Read the model definition and answer for the solid it produces. Units are mm, in the model's axes. Coordinates: 2 decimals unless noted, no trailing zeros. Order: outer loops, then holes, each group sorted by start corner. A loop starts at its lowest first (then second) coordinate and runs counter-clockwise, first axis right, second up.
```python
from build123d import *

# Parameters (mm, degrees)
BOSS_EXTRUDE1_DEPTH             = 2.794
CUT_EXTRUDE1_DEPTH              = 89.482328967
CUT_EXTRUDE1_DEPTH_BACK         = 89.482328967
BOSS_EXTRUDE2_REACH             = 90.482
SKETCH3_W                       = 5.588
SKETCH3_H                       = 12.7
BOSS_EXTRUDE2_DIRECTION_2_REACH = 90.482
BOSS_EXTRUDE3_REACH             = 92.049
SKETCH4_R                       = 2.5273
BOSS_EXTRUDE3_DIRECTION_2_REACH = 92.049
SKETCH6_R                       = 1.2192
CUT_EXTRUDE8_DEPTH              = 91.178457469
CHAMFER1_SIZE                   = 3.175
CUT_EXTRUDE10_DEPTH             = 91.178457469


with BuildPart() as part:
    # Sketch1 → Boss-Extrude1 (new, symmetric)
    with BuildSketch(Plane.XY):
        Polygon((-6.06425, 85.600032), (22.225, 85.600032), (22.225, 0), (-22.225, 0), (-22.225, 85.600032), (-11.90625, 85.600032), (-11.90625, 53.850032), (-6.06425, 53.850032), align=None)
    extrude(amount=BOSS_EXTRUDE1_DEPTH, both=True)

    # Sketch2 → Cut-Extrude1 (cut, two sides: drawn at the far end of the back side and taken through both)
    with BuildSketch(Plane.XY.offset(-CUT_EXTRUDE1_DEPTH_BACK)):
        Polygon((-22.225, 27.78125), (-16.66875, 27.78125), (-16.66875, 30.1625), (-11.90625, 30.1625), (-11.90625, 27.78125), (-6.35, 27.78125), (-6.35, 23.01875), (-11.90625, 23.01875), (-11.90625, 20.6375), (-16.66875, 20.6375), (-16.66875, 23.01875), (-22.225, 23.01875), align=None)
        Polygon((22.225, 27.78125), (16.66875, 27.78125), (16.66875, 30.1625), (11.90625, 30.1625), (11.90625, 27.78125), (6.35, 27.78125), (6.35, 23.01875), (11.90625, 23.01875), (11.90625, 20.6375), (16.66875, 20.6375), (16.66875, 23.01875), (22.225, 23.01875), align=None)
    extrude(amount=CUT_EXTRUDE1_DEPTH + CUT_EXTRUDE1_DEPTH_BACK, mode=Mode.SUBTRACT)

    # Boss-Extrude2: up to this face of the body (flat: up to its plane)
    boss_extrude2_end = Plane(part.part.faces().sort_by_distance((0.486906513, 42.340229634, 2.794))[0])
    # Sketch3 → Boss-Extrude2 (add, up to the picked face)
    with BuildSketch(Plane.XY, mode=Mode.PRIVATE) as boss_extrude2_sk1:
        with Locations((-25.019, 14.208252)):
            Rectangle(SKETCH3_W, SKETCH3_H)
    boss_extrude2_tool1 = split(extrude(boss_extrude2_sk1.sketch, amount=BOSS_EXTRUDE2_REACH, mode=Mode.PRIVATE), bisect_by=boss_extrude2_end, keep=Keep.BOTH, mode=Mode.PRIVATE)
    # Sketch3 → Boss-Extrude2 (add, up to the picked face)
    with BuildSketch(Plane.XY, mode=Mode.PRIVATE) as boss_extrude2_sk2:
        with Locations((25.019, 14.208252)):
            Rectangle(SKETCH3_W, SKETCH3_H)
    boss_extrude2_tool2 = split(extrude(boss_extrude2_sk2.sketch, amount=BOSS_EXTRUDE2_REACH, mode=Mode.PRIVATE), bisect_by=boss_extrude2_end, keep=Keep.BOTH, mode=Mode.PRIVATE)
    # Sketch3 → Boss-Extrude2 (add, up to the picked face)
    with BuildSketch(Plane.XY, mode=Mode.PRIVATE) as boss_extrude2_sk3:
        with Locations((-25.019, 36.591748)):
            Rectangle(SKETCH3_W, SKETCH3_H)
    boss_extrude2_tool3 = split(extrude(boss_extrude2_sk3.sketch, amount=BOSS_EXTRUDE2_REACH, mode=Mode.PRIVATE), bisect_by=boss_extrude2_end, keep=Keep.BOTH, mode=Mode.PRIVATE)
    # Sketch3 → Boss-Extrude2 (add, up to the picked face)
    with BuildSketch(Plane.XY, mode=Mode.PRIVATE) as boss_extrude2_sk4:
        with Locations((25.019, 36.591748)):
            Rectangle(SKETCH3_W, SKETCH3_H)
    boss_extrude2_tool4 = split(extrude(boss_extrude2_sk4.sketch, amount=BOSS_EXTRUDE2_REACH, mode=Mode.PRIVATE), bisect_by=boss_extrude2_end, keep=Keep.BOTH, mode=Mode.PRIVATE)
    add(boss_extrude2_tool1.solids().sort_by(Axis((-25.019, 14.208252, 0), (0, 0, 1)))[0])
    add(boss_extrude2_tool2.solids().sort_by(Axis((25.019, 14.208252, 0), (0, 0, 1)))[0])
    add(boss_extrude2_tool3.solids().sort_by(Axis((-25.019, 36.591748, 0), (0, 0, 1)))[0])
    add(boss_extrude2_tool4.solids().sort_by(Axis((25.019, 36.591748, 0), (0, 0, 1)))[0])

    # Boss-Extrude2 direction 2: up to this face of the body (flat: up to its plane)
    boss_extrude2_direction_2_end = Plane(part.part.faces().sort_by_distance((0.486906513, 42.340229634, -2.794))[0])
    # Sketch3 → Boss-Extrude2 direction 2 (add, up to the picked face)
    with BuildSketch(Plane.XY, mode=Mode.PRIVATE) as boss_extrude2_direction_2_sk1:
        with Locations((-25.019, 14.208252)):
            Rectangle(SKETCH3_W, SKETCH3_H)
    boss_extrude2_direction_2_tool1 = split(extrude(boss_extrude2_direction_2_sk1.sketch, amount=-BOSS_EXTRUDE2_DIRECTION_2_REACH, mode=Mode.PRIVATE), bisect_by=boss_extrude2_direction_2_end, keep=Keep.BOTH, mode=Mode.PRIVATE)
    # Sketch3 → Boss-Extrude2 direction 2 (add, up to the picked face)
    with BuildSketch(Plane.XY, mode=Mode.PRIVATE) as boss_extrude2_direction_2_sk2:
        with Locations((25.019, 14.208252)):
            Rectangle(SKETCH3_W, SKETCH3_H)
    boss_extrude2_direction_2_tool2 = split(extrude(boss_extrude2_direction_2_sk2.sketch, amount=-BOSS_EXTRUDE2_DIRECTION_2_REACH, mode=Mode.PRIVATE), bisect_by=boss_extrude2_direction_2_end, keep=Keep.BOTH, mode=Mode.PRIVATE)
    # Sketch3 → Boss-Extrude2 direction 2 (add, up to the picked face)
    with BuildSketch(Plane.XY, mode=Mode.PRIVATE) as boss_extrude2_direction_2_sk3:
        with Locations((-25.019, 36.591748)):
            Rectangle(SKETCH3_W, SKETCH3_H)
    boss_extrude2_direction_2_tool3 = split(extrude(boss_extrude2_direction_2_sk3.sketch, amount=-BOSS_EXTRUDE2_DIRECTION_2_REACH, mode=Mode.PRIVATE), bisect_by=boss_extrude2_direction_2_end, keep=Keep.BOTH, mode=Mode.PRIVATE)
    # Sketch3 → Boss-Extrude2 direction 2 (add, up to the picked face)
    with BuildSketch(Plane.XY, mode=Mode.PRIVATE) as boss_extrude2_direction_2_sk4:
        with Locations((25.019, 36.591748)):
            Rectangle(SKETCH3_W, SKETCH3_H)
    boss_extrude2_direction_2_tool4 = split(extrude(boss_extrude2_direction_2_sk4.sketch, amount=-BOSS_EXTRUDE2_DIRECTION_2_REACH, mode=Mode.PRIVATE), bisect_by=boss_extrude2_direction_2_end, keep=Keep.BOTH, mode=Mode.PRIVATE)
    add(boss_extrude2_direction_2_tool1.solids().sort_by(Axis((-25.019, 14.208252, 0), (0, 0, -1)))[0])
    add(boss_extrude2_direction_2_tool2.solids().sort_by(Axis((25.019, 14.208252, 0), (0, 0, -1)))[0])
    add(boss_extrude2_direction_2_tool3.solids().sort_by(Axis((-25.019, 36.591748, 0), (0, 0, -1)))[0])
    add(boss_extrude2_direction_2_tool4.solids().sort_by(Axis((25.019, 36.591748, 0), (0, 0, -1)))[0])

    # Boss-Extrude3: up to this face of the body (flat: up to its plane)
    boss_extrude3_end = Plane(part.part.faces().sort_by_distance((0.449618089, 41.042907789, 2.794))[0])
    # Sketch4 → Boss-Extrude3 (add, up to the picked face)
    with BuildSketch(Plane.XY, mode=Mode.PRIVATE) as boss_extrude3_sk1:
        with BuildLine():
            Line((-22.225, 0), (22.225, 0))
            Line((22.225, 0), (22.225, -18.161))
            ThreePointArc((22.225, -18.161), (0, -50.720463079), (-22.225, -18.161))
            Line((-22.225, -18.161), (-22.225, 0))
        make_face()
        with Locations(Location((0, -26.855369585, 0), (0, 0, 180))):
            Circle(SKETCH4_R, mode=Mode.SUBTRACT)
    boss_extrude3_tool1 = split(extrude(boss_extrude3_sk1.sketch, amount=BOSS_EXTRUDE3_REACH, mode=Mode.PRIVATE), bisect_by=boss_extrude3_end, keep=Keep.BOTH, mode=Mode.PRIVATE)
    add(boss_extrude3_tool1.solids().sort_by(Axis((0, -23.48752, 0), (0, 0, 1)))[0])

    # Boss-Extrude3 direction 2: up to this face of the body (flat: up to its plane)
    boss_extrude3_direction_2_end = Plane(part.part.faces().sort_by_distance((0.449618089, 41.042907789, -2.794))[0])
    # Sketch4 → Boss-Extrude3 direction 2 (add, up to the picked face)
    with BuildSketch(Plane.XY, mode=Mode.PRIVATE) as boss_extrude3_direction_2_sk1:
        with BuildLine():
            Line((-22.225, 0), (22.225, 0))
            Line((22.225, 0), (22.225, -18.161))
            ThreePointArc((22.225, -18.161), (0, -50.720463079), (-22.225, -18.161))
            Line((-22.225, -18.161), (-22.225, 0))
        make_face()
        with Locations(Location((0, -26.855369585, 0), (0, 0, 180))):
            Circle(SKETCH4_R, mode=Mode.SUBTRACT)
    boss_extrude3_direction_2_tool1 = split(extrude(boss_extrude3_direction_2_sk1.sketch, amount=-BOSS_EXTRUDE3_DIRECTION_2_REACH, mode=Mode.PRIVATE), bisect_by=boss_extrude3_direction_2_end, keep=Keep.BOTH, mode=Mode.PRIVATE)
    add(boss_extrude3_direction_2_tool1.solids().sort_by(Axis((0, -23.48752, 0), (0, 0, -1)))[0])

    # Sketch6 → Cut-Extrude8 (cut, through all)
    with BuildSketch(Plane.XY.offset(2.794)):
        with Locations((-15.875, -26.855369585)):
            Circle(SKETCH6_R)
        with Locations((-15.334072492, -22.746617244)):
            Circle(SKETCH6_R)
        with Locations((-13.748153285, -18.917869585)):
            Circle(SKETCH6_R)
        with Locations((-11.225320151, -15.630049433)):
            Circle(SKETCH6_R)
        with Locations((-11.225320151, -38.080689736)):
            Circle(SKETCH6_R)
        with Locations((-13.748153285, -34.792869585)):
            Circle(SKETCH6_R)
        with Locations((-15.334072492, -30.964121926)):
            Circle(SKETCH6_R)
    extrude(amount=-CUT_EXTRUDE8_DEPTH, mode=Mode.SUBTRACT)

    # Chamfer1
    chamfer1_edges = [part.edges().sort_by_distance(p)[0] for p in [
        (-11.90625, 85.600032, 0),
        (-6.06425, 85.600032, 0),
    ]]
    chamfer(chamfer1_edges, length=CHAMFER1_SIZE)

    # Sketch8 → Cut-Extrude10 (cut, through all)
    with BuildSketch(Plane.XY.offset(2.794)):
        with BuildLine():
            Line((5.129422909, 52.414421713), (12.749422909, 52.414421713))
            ThreePointArc((12.749422909, 52.414421713), (19.099422909, 46.064421713), (12.749422909, 39.714421713))
            Line((12.749422909, 39.714421713), (5.129422909, 39.714421713))
            ThreePointArc((5.129422909, 39.714421713), (-1.220577091, 46.064421713), (5.129422909, 52.414421713))
        make_face()
    extrude(amount=-CUT_EXTRUDE10_DEPTH, mode=Mode.SUBTRACT)


solid = part.part
```
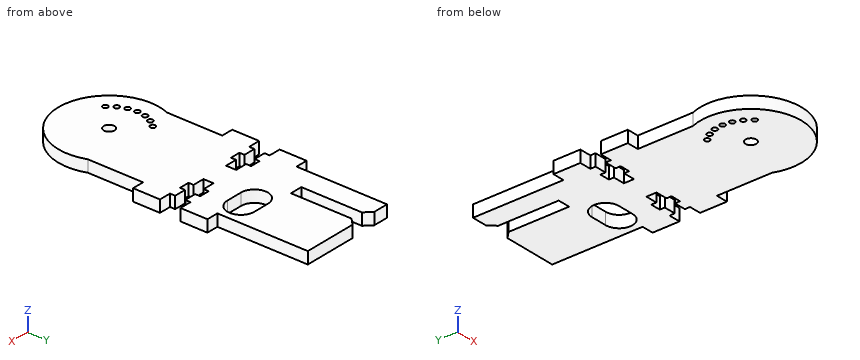
1) Flat-ended cylindrical pins translate along their axes: pin 1 Ø3 at (y, z) = (-0.5, -1) entering from -X (3 decimals); pin 2 Ø3 at (y, z) = (-20.5, 1.5) entering from -X; pin 3 Ø0.7 at (y, z) = (28.5, -1) entering from +X (3 decimals). Find the tip coordinate at first contact, or state that the pin passes through.
A:
pin 1: stops at x = -22.225
pin 2: stops at x = -23.37
pin 3: stops at x = 22.225
2) A cutting plane is placed at D-D, the plane y = -12. Determine the outline of the cut face in (x, z) (3 decimals).
A:
outline: (-22.225, -2.794) - (22.225, -2.794) - (22.225, 2.794) - (-22.225, 2.794) - close
3) A cutting plane is placed at B-B, the plane x = 14. Determine the outline of the cut face in (y, z), and give its area (3 significant figures).
A:
outline: (-46.18, -2.79) - (20.64, -2.79) - (20.64, 2.79) - (-46.18, 2.79) - close; (30.16, -2.79) - (39.84, -2.79) - (39.84, 2.79) - (30.16, 2.79) - close; (52.29, -2.79) - (85.6, -2.79) - (85.6, 2.79) - (52.29, 2.79) - close
area: 614 mm2
4) A cutting plane is placed at A-A, the plane y = 70. Determine the outline of the cut face in (x, z) (3 decimals).
A:
outline: (-22.225, -2.794) - (-11.906, -2.794) - (-11.906, 2.794) - (-22.225, 2.794) - close; (-6.064, -2.794) - (22.225, -2.794) - (22.225, 2.794) - (-6.064, 2.794) - close
5) A cutting plane is placed at C-C, the plane x = 0. Determine the outline of the cut face in (y, z).
A:
outline: (-50.72, -2.79) - (-29.38, -2.79) - (-29.38, 2.79) - (-50.72, 2.79) - close; (-24.33, -2.79) - (42.32, -2.79) - (42.32, 2.79) - (-24.33, 2.79) - close; (49.81, -2.79) - (85.6, -2.79) - (85.6, 2.79) - (49.81, 2.79) - close
6) Straight lines are drawn through the part: line 1 (Y direction, x = 25, z = 0.8); line 2 (Y direction, x = 12, z = 1.45); line 3 (Y direction, x = 11, z = -1.7). For each, find the intervals that lie inside material, in ascending order.
A:
line 1: y = 7.86 to 20.56, 30.24 to 42.94
line 2: y = -47.48 to 20.64, 30.16 to 39.71, 52.41 to 85.6
line 3: y = -48.03 to 23.02, 27.78 to 39.71, 52.41 to 85.6
